Read the model definition and answer for the solid it produces. Units are mm, in the model's axes. A direction names the side the tool comes from. Give positions to 0.01 mm unless a question says otherwise; leave off trailing zeros. Write each loop counter-clockwise with the first axis right and the second up, starting at its lowest first coordinate (ties: lowest second). Pieces come first, ordered by that corner, then holes. Notation, with made-up numbers: (9.25, 3.25) - (18.25, 3.25) arc R12 cw to (18.25, 24.25) - close; hole circle Ø10 at (18, 78.25). An arc over 180 degrees is marked (long way). Answer as a JSON object with one key per item and string values. Group by question number.
```python
from build123d import *

# Parameters (mm, degrees)
PAD_DEPTH            = 10
PAD002_DEPTH         = 26.85
POCKET_DEPTH         = 0.001
POCKET_DEPTH_BACK    = -14.001
SKETCH004_W          = 82.61631
SKETCH004_H          = 35.698411
SKETCH004_W_2        = 63.407177
SKETCH004_H_2        = 9.483432
POCKET001_DEPTH      = 14.593528
POCKET001_DEPTH_BACK = -14.593528


with BuildPart() as part:
    # Sketch → Pad (new body)
    with BuildSketch(Plane.XY):
        Polygon((16.85, 0), (8.425, 14.592528), (-8.425, 14.592528), (-16.85, 0), (-8.425, -14.592528), (8.425, -14.592528), align=None)
        Polygon((10.85, 0), (5.425, 9.396376), (-5.425, 9.396376), (-10.85, 0), (-5.425, -9.396376), (5.425, -9.396376), align=None, mode=Mode.SUBTRACT)
    extrude(amount=PAD_DEPTH)

    # Sketch002 → Pad002 (join, symmetric)
    with BuildSketch(Plane.YZ):
        with BuildLine():
            ThreePointArc((4, 10), (0, 14), (-4, 10))
            Line((-4, 10), (-4, 0))
            Line((-4, 0), (4, 0))
            Line((4, 0), (4, 10))
        make_face()
    extrude(amount=PAD002_DEPTH, both=True)

    # Sketch003 → Pocket (cut, two sides)
    with BuildSketch(Plane.XY) as pocket_sk:
        Polygon((10.85, 0), (5.425, 9.396376), (-5.425, 9.396376), (-10.85, 0), (-5.425, -9.396376), (5.425, -9.396376), align=None)
    extrude(amount=-POCKET_DEPTH, mode=Mode.SUBTRACT)
    extrude(pocket_sk.sketch, amount=-POCKET_DEPTH_BACK, mode=Mode.SUBTRACT)

    # Sketch004 → Pocket001 (cut, two sides)
    with BuildSketch(Plane.XZ) as pocket001_sk:
        with Locations((0.841957, 8.089457)):
            Rectangle(SKETCH004_W, SKETCH004_H)
        with Locations((-0.35511, 2.858284)):
            Rectangle(SKETCH004_W_2, SKETCH004_H_2, mode=Mode.SUBTRACT)
    extrude(amount=-POCKET001_DEPTH, mode=Mode.SUBTRACT)
    extrude(pocket001_sk.sketch, amount=-POCKET001_DEPTH_BACK, mode=Mode.SUBTRACT)


solid = part.part
```
1) Flat-ended cylindrical pins translate along their axes: pin 1 Ø2.5 at (x, z) = (-23, 4.5) entering from -Y; pin 2 Ø4 at (x, z) = (19, 5) entering from +Y; pin 3 Ø1 at (y, z) = (10.5, 6) entering from +X. Find the tip coordinate at first contact, or state that the pin passes through.
2) Find section B-B, the plane z = 1.75. Write down the section's boundary in (x, y) (3 decimals), and give its area (3 significant figures).
3) Which of the six approach directions +Z, -Z, +X, -X, +Y, -Y give full straight-line access (tool end or side, diameter ignored) to faces 4 (the flat face through (8.175, 4.632, 3.747)), 5 (the flat face through (21, -4, 4)), 6 (the flat face through (-21, 4, 4))?
4) Find the intervals of material crossed by line 1 (Y direction, x = 5, z = 3.75); line 2 (X direction, y = -3.25, z = 5.5); line 3 (Y direction, x = 19.5, z = 1.25), in increasing order. Write a range as [from, to].
5) Find section D-D, the plane x = 19. Write down the section's boundary in (y, z), and give its area (3 significant figures).
6) Find section C-C, the plane y = 8.75. Write down the section's boundary in (x, z).
7) For a pull along X with two mould halves and no side action, classify faces 1 (the flat face through (21, 4, 4)), 2 (the flat face through (-8.1, 4.76, 3.75)), 3 (the flat face through (-11.44, 9.37, 3.75)) as released by +X, released by -X, zero draft, split by the parting line, or undercut.
8) Find section A-A, the plane x = -3.5. Write down the section's boundary in (y, z), and give its area (3 significant figures).
Values follow:
{
 "1": {"pin 1": "stops at y = -4", "pin 2": "stops at y = 4", "pin 3": "stops at x = 11.08"},
 "2": {"outline": "(-26.85, -4) - (-14.541, -4) - (-8.425, -14.593) - (8.425, -14.593) - (14.541, -4) - (26.85, -4) - (26.85, 4) - (14.541, 4) - (8.425, 14.593) - (-8.425, 14.593) - (-14.541, 4) - (-26.85, 4) - close; hole (-10.85, 0) - (-5.425, -9.396) - (5.425, -9.396) - (10.85, 0) - (5.425, 9.396) - (-5.425, 9.396) - close", "area": "610 mm2"},
 "3": {"face 4": "+Z, -Z", "face 5": "+Z, -Z, +X, -Y", "face 6": "+Z, -Z, -X, +Y"},
 "4": {"line 1": "y = [-14.59, -9.4], [9.4, 14.59]", "line 2": "x = [-26.85, -8.97], [8.97, 26.85]", "line 3": "y = [-4, 4]"},
 "5": {"outline": "(-4, 0) - (4, 0) - (4, 7.6) - (-4, 7.6) - close", "area": "60.8 mm2"},
 "6": {"outline": "(-11.8, 0) - (-5.8, 0) - (-5.8, 7.6) - (-11.8, 7.6) - close; (5.8, 0) - (11.8, 0) - (11.8, 7.6) - (5.8, 7.6) - close"},
 "7": {"face 1": "zero draft", "face 2": "undercut", "face 3": "released by -X"},
 "8": {"outline": "(-14.59, 0) - (-9.4, 0) - (-9.4, 7.6) - (-14.59, 7.6) - close; (9.4, 0) - (14.59, 0) - (14.59, 7.6) - (9.4, 7.6) - close", "area": "79.0 mm2"}
}
